```python
from build123d import *

# Parameters (mm, degrees)
SKETCH2_W           = 2.5
SKETCH2_H           = 7
SKETCH2_W_2         = 32
SKETCH2_H_2         = 10
SKETCH2_W_3         = 10
SKETCH4_W           = 3.5
SKETCH4_H           = 22
CUT_EXTRUDE1_DEPTH  = 32
CUT_EXTRUDE2_DEPTH  = 2.5
SKETCH6_R           = 2
BOSS_EXTRUDE1_DEPTH = 12
SKETCH7_W           = 4
SKETCH7_H           = 2
CUT_EXTRUDE3_DEPTH  = 8


with BuildPart() as part:
    # Sketch2 → Revolve1 (revolve)
    with BuildSketch(Plane(origin=(0, 0, 0), x_dir=(0, 0, -1), z_dir=(1, 0, 0)), mode=Mode.PRIVATE) as revolve1_sk:
        with Locations((-19.25, 3.5)):
            Rectangle(SKETCH2_W, SKETCH2_H)
        Polygon((-18, 0), (0, 0), (0, 10), (0, 11), (-18, 11), (-18, 7), align=None)
        with Locations((16, 5)):
            Rectangle(SKETCH2_W_2, SKETCH2_H_2)
        with Locations((37, 5)):
            Rectangle(SKETCH2_W_3, SKETCH2_H_2)
    revolve(revolve1_sk.sketch.rotate(Axis((0, 0, 51.295546559), (0, 0, -1)), 90), axis=Axis((0, 0, 51.295546559), (0, 0, -1)))

    # Sketch4 → Cut-Extrude1 (cut)
    with BuildSketch(Plane(origin=(0, 0, 0), x_dir=(-1, 0, 0), z_dir=(0, 0, -1))):
        with Locations((-9.25, 0)):
            Rectangle(SKETCH4_W, SKETCH4_H)
        with Locations((9.25, 0)):
            Rectangle(SKETCH4_W, SKETCH4_H)
    extrude(amount=CUT_EXTRUDE1_DEPTH, mode=Mode.SUBTRACT)

    # Sketch5 → Cut-Extrude2 (cut)
    with BuildSketch(Plane.XY.offset(20.5)):
        Polygon((-9.192388155, 0.707106781), (0.707106781, -9.192388155), (-2.828427125, -12.727922061), (-12.727922061, -2.828427125), align=None)
        Polygon((-0.707106781, 9.192388155), (9.192388155, -0.707106781), (12.727922061, 2.828427125), (2.828427125, 12.727922061), align=None)
    extrude(amount=-CUT_EXTRUDE2_DEPTH, mode=Mode.SUBTRACT)

    # Sketch6 → Boss-Extrude1 (add)
    with BuildSketch(Plane.XY.offset(20.5)):
        Circle(SKETCH6_R)
    extrude(amount=BOSS_EXTRUDE1_DEPTH)

    # Sketch7 → Cut-Extrude3 (cut)
    with BuildSketch(Plane.XY.offset(32.5)):
        with Locations((0, 2)):
            Rectangle(SKETCH7_W, SKETCH7_H)
    extrude(amount=-CUT_EXTRUDE3_DEPTH, mode=Mode.SUBTRACT)


solid = part.part
```
Geometry check sheet. Reference: the model listing, model coordinates, mm. A direction names the side the tool comes from. Give positions to 0.01 mm unless a question says otherwise; leave off trailing zeros. Order: outer loops, then holes, each group sorted by start corner. A loop starts at its lowest first (then second) coordinate and runs counter-clockwise, first axis right, second up.
1. Section check B-B, the plane y = 0. Enter the section's corners in (x, z).
2. Section check A-A, the plane x = 0. Enter the section's corners in (y, z), and give its area (3 significant figures).
3. Thickness scan on L1, parallel to Z at x = -7.75, y = 0.75; L2, parallel to Z at x = -6, y = 5.5; L3, parallel to Z at x = 4, y = 3. Record the ranges inside material, lowest first.
4. Section check D-D, the plane y = -8.75. Enter the section's corners in (x, z).
5. Gauge pin test, flat ends, axial feed: pin 1 Ø6 at (x, z) = (-8, 5.5) entering from +Y; pin 2 Ø3 at (x, y) = (8, -1.5) entering from +Z; pin 3 Ø3 at (x, z) = (0, 30) entering from +Y. Record the tip position at first contact, or that the pin passes through.
6. Access from +Z, -Z, +X, -X, +Y, -Y to the whole of each face (thin tool, end or side, straight path). Record for faces 5 (the face through (4.207, 4.278, 19.268)), 6 (the face through (0, -2, 26)), 7 (the face through (-7.5, 0, -16)), 8 (the face through (-8, 0, 0)), 9 (the face through (-4.278, -4.207, 19.268)).
7. Section check C-C, the plane z = -15. Enter the section's corners in (x, y).
8. Release check for a two-part mould opening along Z. For faces 1 (the face through (7.5, 0, -16)), 2 (the face through (8, 0, -32)), 3 (the face through (-5, 4.9, 19.2)), 4 (the face through (0, 0, -42)) record: pulls with the +Z half, pulls with the -Z half, needs draft (parallel to the pull), parting line crosses it, or undercut.
Values follow:
1. outline: (-11, 0) - (-7.5, 0) - (-7.5, -32) - (-10, -32) - (-10, -42) - (10, -42) - (10, -32) - (7.5, -32) - (7.5, 0) - (11, 0) - (11, 18) - (7, 18) - (7, 20.5) - (2, 20.5) - (2, 32.5) - (-2, 32.5) - (-2, 20.5) - (-7, 20.5) - (-7, 18) - (-11, 18) - close
2. outline: (-11, 0) - (-10, 0) - (-10, -42) - (10, -42) - (10, 0) - (11, 0) - (11, 18) - (7, 18) - (7, 20.5) - (2, 20.5) - (2, 24.5) - (1, 24.5) - (1, 32.5) - (-2, 32.5) - (-2, 20.5) - (-7, 20.5) - (-7, 18) - (-11, 18) - close
2. area: 1,310 mm2
3. L1: z = -42 to -32, 0 to 18
3. L2: z = -42 to 18
3. L3: z = -42 to 20.5
4. outline: (-6.67, 0) - (-4.84, 0) - (-4.84, -42) - (4.84, -42) - (4.84, 0) - (6.67, 0) - (6.67, 18) - (-6.67, 18) - close
5. pin 1: stops at y = 9.8
5. pin 2: stops at z = 20.5
5. pin 3: stops at y = 1
6. face 5: +Z, +X, +Y
6. face 6: +Z
6. face 7: -X, +Y, -Y
6. face 8: none
6. face 9: +Z, -X, -Y
7. outline: (-7.5, -6.61) arc R10 ccw to (7.5, -6.61) - (7.5, 6.61) arc R10 ccw to (-7.5, 6.61) - close
8. face 1: undercut
8. face 2: undercut
8. face 3: needs draft
8. face 4: pulls with the -Z half
